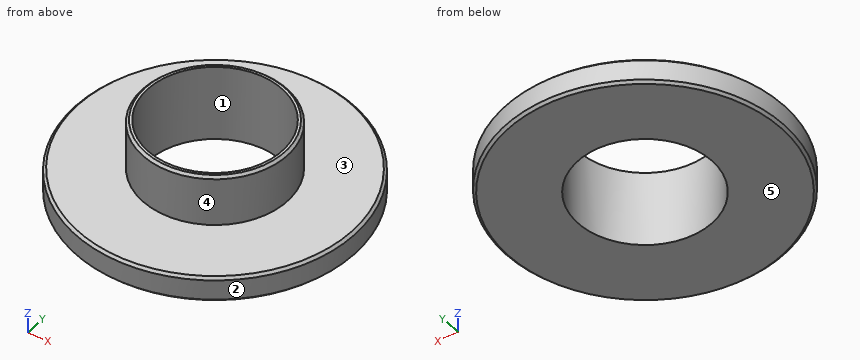
```python
from build123d import *

# Parameters (mm, degrees)
F2_SIZE = 1
F3_SIZE = 1


with BuildPart() as f1:
    # F0 (on Front) → F1 (revolve)
    with BuildSketch(Plane.XZ):
        Polygon((-28.5, 10), (-55, 10), (-55, 0), (-26.5, 0), (-26.5, 30), (-28.5, 30), align=None)
    revolve(axis=Axis((0, 0, 60.018875), (0, 0, -1)))

    # F2
    f2_edges = [f1.edges().sort_by_distance(p)[0] for p in [
        (55, 0, 10),
    ]]
    chamfer(f2_edges, length=F2_SIZE)

    # F3
    f3_edges = [f1.edges().sort_by_distance(p)[0] for p in [
        (28.5, 0, 30),
        (55, 0, 0),
    ]]
    chamfer(f3_edges, length=F3_SIZE)


solid = f1.part
```
Check sheet for the modelled part. Datum: model origin and axes. Units: mm. Face numbers are marked on the shaded views. A direction names the side the tool comes from. Round coordinates to 2 decimals unless told otherwise and drop trailing zeros. Loops run counter-clockwise (first coordinate to the right, second up) from the corner with the lowest first, then second, coordinate; pieces in that order, holes last. Notation, with made-up numbers: M 79.25,-30.5 L 123.25,-30.5 A25 cw 123.25,-15.5 Z; hole C -38.5,-19.5 d3. An arc over 180 degrees is marked long. Answer as a JSON object with one key per item and string values.
1. Scan lines: line 1 (Y direction, x = 0, z = 11.25); line 2 (Z direction, x = -27.5, y = 25); line 3 (Y direction, x = 0, z = 8.5). Record each from-to range of solid material in increasing order.
Reply:
{"line 1": "y = -28.5 to -26.5, 26.5 to 28.5", "line 2": "z = 0 to 10", "line 3": "y = -55 to -26.5, 26.5 to 55"}
2. Section check C-C (z = 27.5). Record the boundary of the cut face in (x, y), plus the area to 3 significant figures.
Reply:
{"outline": "C 0,0 d57; hole C 0,0 d53", "area": "346 mm²"}
3. Section check A-A (x = 0). Record the boundary of the cut face in (y, z), plus the area to 3 significant figures.
Reply:
{"outline": "M -55,1 L -54,0 L -26.5,0 L -26.5,30 L -27.5,30 L -28.5,29 L -28.5,10 L -54,10 L -55,9 Z; M 26.5,0 L 54,0 L 55,1 L 55,9 L 54,10 L 28.5,10 L 28.5,29 L 27.5,30 L 26.5,30 Z", "area": "647 mm²"}
4. Gauge pin test, flat ends, axial feed: P1, Ø1.5, axis at x = -4, y = 40.5, coming from the +Z side; P2, Ø3, axis at x = -6.5, z = 17, coming from the +Y side; P3, Ø12, axis at x = 22.5, z = 7, coming from the -Y side. Record the tip position at first contact, or that the pin passes through.
Reply:
{"P1": "stops at z = 10", "P2": "stops at y = 28.06", "P3": "stops at y = -52.47"}
5. Access from +Z, -Z, +X, -X, +Y, -Y to the whole of each face (thin tool, end or side, straight path). Record for the marked faces 4 and 5.
Reply:
{"face 4": "+Z", "face 5": "-Z, +X, -X, +Y, -Y"}
6. Section check D-D (z = 6.25). Record the boundary of the cut face in (x, y).
Reply:
{"outline": "C 0,0 d110; hole C 0,0 d53"}
7. Mould release check, pull along X, two halves, no side actions. Record for the marked faces 1, 2 and 3: pulls with the +X half, pulls with the -X half, needs draft (parallel to the pull), parting line crosses it, or undercut.
Reply:
{"face 1": "undercut", "face 2": "parting line crosses it", "face 3": "needs draft"}
